```python
from build123d import *

# Parameters (mm, degrees)
F0_R           = 381
F1_DEPTH       = 12.7
F3_D           = 90
F5_D           = 8.8
F5_CSINK_D     = 17.92
F5_CSINK_ANGLE = 90
F7_D           = 76.2


with BuildPart() as f1:
    # F0 (on Top) → F1 (new body)
    with BuildSketch(Plane.XY):
        Circle(F0_R)
    extrude(amount=-F1_DEPTH)

    # F3 (through all)
    with Locations(Plane.XY):
        with Locations((0, 0)):
            Hole(F3_D / 2)

    # F5 (through all)
    with Locations(Plane.XY):
        with Locations((0, 76.2), (65.9911357684, 38.1), (65.9911357684, -38.1), (0, -76.2), (-65.9911357684, -38.1), (-65.9911357684, 38.1)):
            CounterSinkHole(F5_D / 2, F5_CSINK_D / 2, counter_sink_angle=F5_CSINK_ANGLE)

    # F7 (through all)
    with Locations(Plane.XY):
        with Locations((0, 304.8), (304.8, 0), (0, -304.8), (-304.8, 0)):
            Hole(F7_D / 2)


solid = f1.part
```
Could you check a few things on this model? Use its own coordinates, in mm. Round coordinates to 2 decimals unless told otherwise and drop trailing zeros. Loops run counter-clockwise (first coordinate to the right, second up) from the corner with the lowest first, then second, coordinate; pieces in that order, holes last. Notation, with made-up numbers: (23, 44) - (53, 44) arc R18 ccw to (53, 75) - close; hole circle Ø3 at (21, 82). An arc over 180 degrees is marked (long way). Answer in a Markdown table with one row per item. Add a question column.
(1) If we mould it in two halves opening along X, with no side actions, what happens to faces 1 (the face through (-5, -79, -12.7)), 2 (the face through (-302.35, -231.83, -6.26)), 3 (the face through (-64.99, -42.61, -4.34))? For each: pulls with the +X half, pulls with the -X half, needs draft (parallel to the pull), parting line crosses it, or undercut.
(2) If we section it at D-D (z = -10.25): State how many separate pieces and enclosed holes the cut face has, plus the area to 3 significant figures.
(3) If we section it at C-C (y = 0): Please give me the cut outline in (x, z), plus the area to 3 significant figures.
(4) I need wall thicknesses on line 1 along X through (y, z) = (1, -11.75); line 2 along Y through (x, z) = (0, -10.5); line 3 along Y through (x, z) = (66.5, -4.5). Which ranges of each line are inside material? Lowest first, please.
(5) I'm going to push flat-ended pins straight in: pin 1 (1.5 mm diameter, centred on y = -231, z = -6.5, fed in from -X); pin 2 (6 mm diameter, centred on x = -237, z = -1.5, fed in from +Y); pin 3 (10 mm diameter, centred on x = 65.99, y = 38.1, fed in from -Z); pin 4 (5 mm diameter, centred on y = 288, z = -8, fed in from +X). Where does each tip first touch, or does it pass through?
(6) If we section it at A-A (y = -304.8): Please give me the cut outline in (x, z).
Model answer:
| question | item | result |
|---|---|---|
| 1 | face 1 | needs draft |
| 1 | face 2 | parting line crosses it |
| 1 | face 3 | undercut |
| 2 | separate pieces | 1 |
| 2 | enclosed holes | 11 |
| 2 | area | 431,000 mm² |
| 3 | outline | (-381, -12.7) - (-342.9, -12.7) - (-342.9, 0) - (-381, 0) - close; (-266.7, -12.7) - (-45, -12.7) - (-45, 0) - (-266.7, 0) - close; (45, -12.7) - (266.7, -12.7) - (266.7, 0) - (45, 0) - close; (342.9, -12.7) - (381, -12.7) - (381, 0) - (342.9, 0) - close |
| 3 | area | 6,600 mm² |
| 4 | line 1 | x = -381 to -342.89, -266.71 to -44.99, 44.99 to 266.71, 342.89 to 381 |
| 4 | line 2 | y = -381 to -342.9, -266.7 to -80.6, -71.8 to -45, 45 to 71.8, 80.6 to 266.7, 342.9 to 381 |
| 4 | line 3 | y = -375.15 to -42.53, -33.67 to 33.67, 42.53 to 375.15 |
| 5 | pin 1 | stops at x = -303.56 |
| 5 | pin 2 | stops at y = 300.67 |
| 5 | pin 3 | stops at z = -12.7 |
| 5 | pin 4 | stops at x = 252.29 |
| 6 | outline | (-228.6, -12.7) - (-38.1, -12.7) - (-38.1, 0) - (-228.6, 0) - close; (38.1, -12.7) - (228.6, -12.7) - (228.6, 0) - (38.1, 0) - close |
